Could you check a few things on this drawing? It's one solid part, dimensions in mm from its lowest x, y, z. A direction names the side the tool comes from. Round coordinates to 2 decimals unless told otherwise and drop trailing zeros. Loops run counter-clockwise (first coordinate to the right, second up) from the corner with the lowest first, then second, coordinate; pieces in that order, holes last. Notation, with made-up numbers: (-11.5, -39) -> (21.5, -39) arc R23 cw to (21.5, -29) -> close; hole circle Ø3 at (2.25, 74.25). An arc over 180 degrees is marked (long way). Write each question's results on one line, items separated by ' | '.
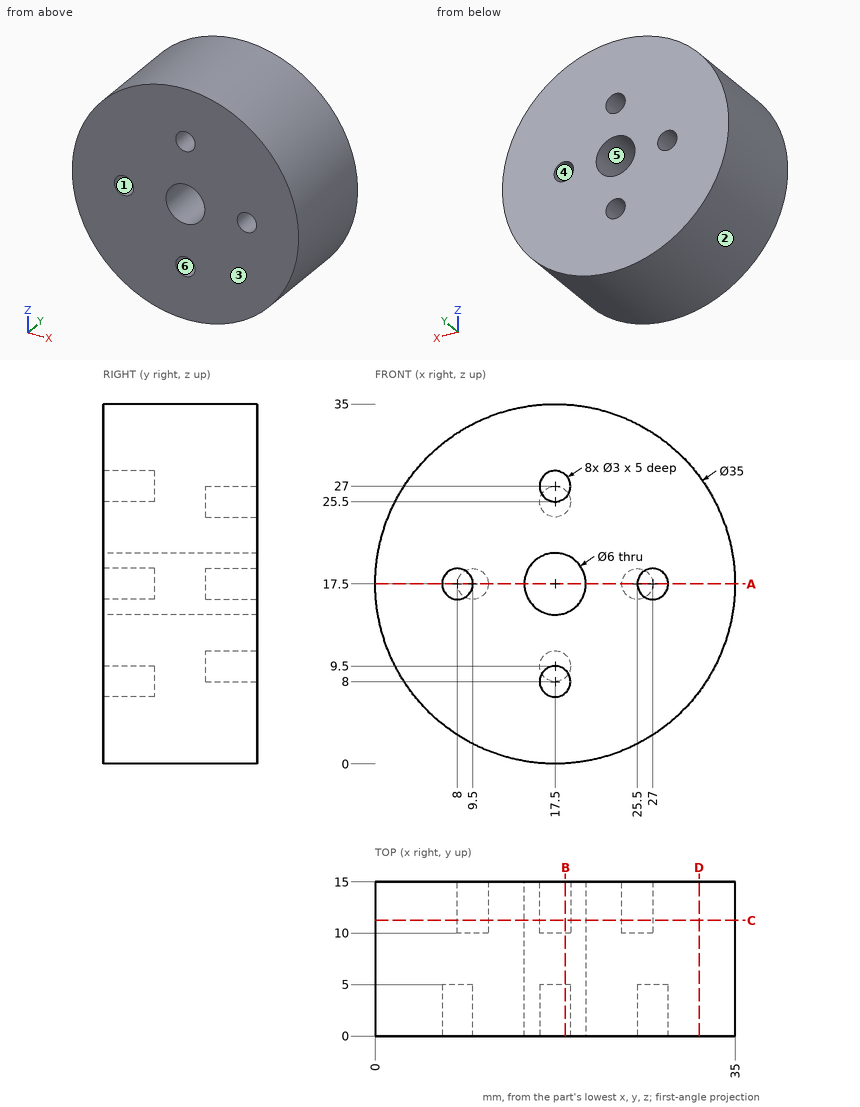
1) For the marked faces 4, 5 and 6, which set-ups out of +Z, -Z, +X, -X, +Y, -Y let a thin tool reach every point of the face, with its end or its side?
Model answer:
face 4: +Y | face 5: +Y, -Y | face 6: -Y
2) I want a section at B-B, the plane x = 18.5. Write out the boundary of the cut face in (y, z), plus the area to 3 significant figures.
Model answer:
outline: (0, 0.03) -> (15, 0.03) -> (15, 8.38) -> (10, 8.38) -> (10, 10.62) -> (15, 10.62) -> (15, 14.67) -> (0, 14.67) -> (0, 9.12) -> (5, 9.12) -> (5, 6.88) -> (0, 6.88) -> close; (0, 20.33) -> (15, 20.33) -> (15, 24.38) -> (10, 24.38) -> (10, 26.62) -> (15, 26.62) -> (15, 34.97) -> (0, 34.97) -> (0, 28.12) -> (5, 28.12) -> (5, 25.88) -> (0, 25.88) -> close | area: 395 mm2
3) If we mould it in two halves opening along Z, with no side actions, what happens to the marked faces 1, 2 and 3? For each: released by +Z, released by -Z, zero draft, split by the parting line, or undercut.
Model answer:
face 1: undercut | face 2: split by the parting line | face 3: zero draft
4) I'm going to push flat-ended pins straight in: pin 1 (1.5 mm diameter, centred on y = 4, z = 15, fed in from +X); pin 2 (1.5 mm diameter, centred on x = 7.5, z = 18, fed in from -Y); pin 3 (2.5 mm diameter, centred on x = 17.5, z = 9.5, fed in from +Y). Where does each tip first touch, or does it pass through?
Model answer:
pin 1: stops at x = 34.91 | pin 2: stops at y = 5 | pin 3: stops at y = 10
5) I want a section at A-A, the plane z = 17.5. Write out the boundary of the cut face in (x, y), plus the area to 3 significant figures.
Model answer:
outline: (0, 0) -> (6.5, 0) -> (6.5, 5) -> (9.5, 5) -> (9.5, 0) -> (14.5, 0) -> (14.5, 15) -> (11, 15) -> (11, 10) -> (8, 10) -> (8, 15) -> (0, 15) -> close; (20.5, 0) -> (25.5, 0) -> (25.5, 5) -> (28.5, 5) -> (28.5, 0) -> (35, 0) -> (35, 15) -> (27, 15) -> (27, 10) -> (24, 10) -> (24, 15) -> (20.5, 15) -> close | area: 375 mm2
6) I want a section at C-C, the plane y = 11.25. Write out the boundary of the cut face in (x, z), plus the area to 3 significant figures.
Model answer:
outline: circle Ø35 at (17.5, 17.5); hole circle Ø3 at (9.5, 17.5); hole circle Ø6 at (17.5, 17.5); hole circle Ø3 at (17.5, 9.5); hole circle Ø3 at (17.5, 25.5); hole circle Ø3 at (25.5, 17.5) | area: 906 mm2
7) I need wall thicknesses on line 1 (X direction, y = 13.9, z = 17.5); line 2 (Z direction, x = 17.5, y = 3.05). Which ranges of each line are inside material? Lowest first, please.
Model answer:
line 1: x = 0 to 8, 11 to 14.5, 20.5 to 24, 27 to 35 | line 2: z = 0 to 6.5, 9.5 to 14.5, 20.5 to 25.5, 28.5 to 35
8) I want a section at D-D, the plane x = 31.5. Write out the boundary of the cut face in (y, z), plus the area to 3 significant figures.
Model answer:
outline: (0, 7) -> (15, 7) -> (15, 28) -> (0, 28) -> close | area: 315 mm2
